The figure shows three views and two pictorial views of one solid part (mm, origin at its lowest corner). Answer the questions. A direction names the side the tool comes from. Coordinates: 2 decimals unless noted, no trailing zeros. Order: outer loops, then holes, each group sorted by start corner. A loop starts at its lowest first (then second) coordinate and runs counter-clockwise, first axis right, second up. Notation, with made-up numbers: (34, 49) -> (74, 49) arc R33 ccw to (74, 84) -> close; hole circle Ø6 at (-4.5, -16). An arc over 180 degrees is marked (long way). Return JSON: item names as keys, results as strings.
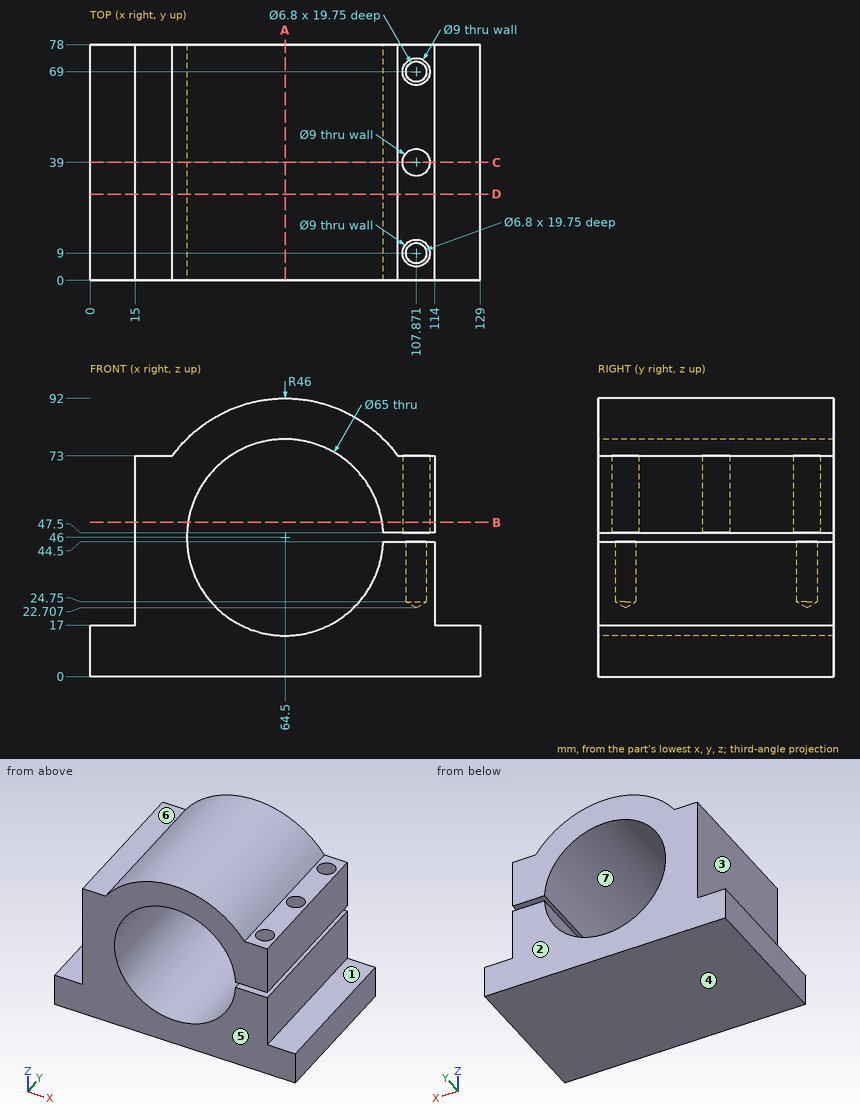
Item 1: Which of the six approach directions +Z, -Z, +X, -X, +Y, -Y give full straight-line access (tool end or side, diameter ignored) to the marked faces 1, 2 and 3?
Answer list:
{"face 1": "+Z, +X, +Y, -Y", "face 2": "+Z, -Z, +X, -X, +Y", "face 3": "+Z, -X, +Y, -Y"}
Item 2: Find the intervals of material crossed by probe 1 along Z at (x, y) = (64, 36); probe 2 along Y at (x, z) = (108.5, 44); probe 3 along Z at (x, y) = (110, 25.5), in increasing order.
Answer list:
{"probe 1": "0 to 13.5, 78.5 to 92", "probe 2": "0 to 5.66, 12.34 to 65.66, 72.34 to 78", "probe 3": "0 to 44.5, 47.5 to 73"}
Item 3: Determine the mould class of the marked faces 4, 5, 6 and 7 for opening direction Z: pulls with the +Z half, pulls with the -Z half, needs draft (parallel to the pull), parting line crosses it, or undercut.
Answer list:
{"face 4": "pulls with the -Z half", "face 5": "needs draft", "face 6": "pulls with the +Z half", "face 7": "undercut"}
Item 4: The part is cut by section C-C on y = 39. Determine the outline of the cut face in (x, z) (1 decimal).
Answer list:
{"outline": "(0, 0) -> (129, 0) -> (129, 17) -> (114, 17) -> (114, 44.5) -> (97, 44.5) arc R32.5 cw (long way) to (97, 47.5) -> (103.4, 47.5) -> (103.4, 73) -> (101.7, 73) arc R46 ccw to (27.3, 73) -> (15, 73) -> (15, 17) -> (0, 17) -> close; (112.4, 47.5) -> (114, 47.5) -> (114, 73) -> (112.4, 73) -> close"}
Item 5: The part is cut by section A-A on x = 64.5. Determine the outline of the cut face in (y, z), plus the area to 3 significant figures.
Answer list:
{"outline": "(0, 0) -> (78, 0) -> (78, 13.5) -> (0, 13.5) -> close; (0, 78.5) -> (78, 78.5) -> (78, 92) -> (0, 92) -> close", "area": "2,110 mm2"}
Item 6: Flat-ended cylindrical pins translate along their axes: pin 1 (2 mm diameter, centred on y = 69, z = 18.5, fed in from -X); pin 2 (10 mm diameter, centred on x = 73.5, y = 50, fed in from +Z); pin 3 (12 mm diameter, centred on x = 122.5, y = 41, fed in from +Z). Find the tip coordinate at first contact, or state that the pin passes through.
Answer list:
{"pin 1": "x = 15", "pin 2": "z = 91.83", "pin 3": "z = 17"}
Item 7: The part is cut by section D-D on y = 28.5. Determine the outline of the cut face in (x, z) (1 decimal), plus the area to 3 significant figures.
Answer list:
{"outline": "(0, 0) -> (129, 0) -> (129, 17) -> (114, 17) -> (114, 44.5) -> (97, 44.5) arc R32.5 cw (long way) to (97, 47.5) -> (114, 47.5) -> (114, 73) -> (101.7, 73) arc R46 ccw to (27.3, 73) -> (15, 73) -> (15, 17) -> (0, 17) -> close", "area": "5,360 mm2"}
Item 8: The part is cut by section B-B on z = 51. Determine the outline of the cut face in (x, y), plus the area to 3 significant figures.
Answer list:
{"outline": "(15, 0) -> (32.39, 0) -> (32.39, 78) -> (15, 78) -> close; (96.61, 0) -> (114, 0) -> (114, 78) -> (96.61, 78) -> close; hole circle Ø9 at (107.87, 9); hole circle Ø9 at (107.87, 39); hole circle Ø9 at (107.87, 69)", "area": "2,520 mm2"}
